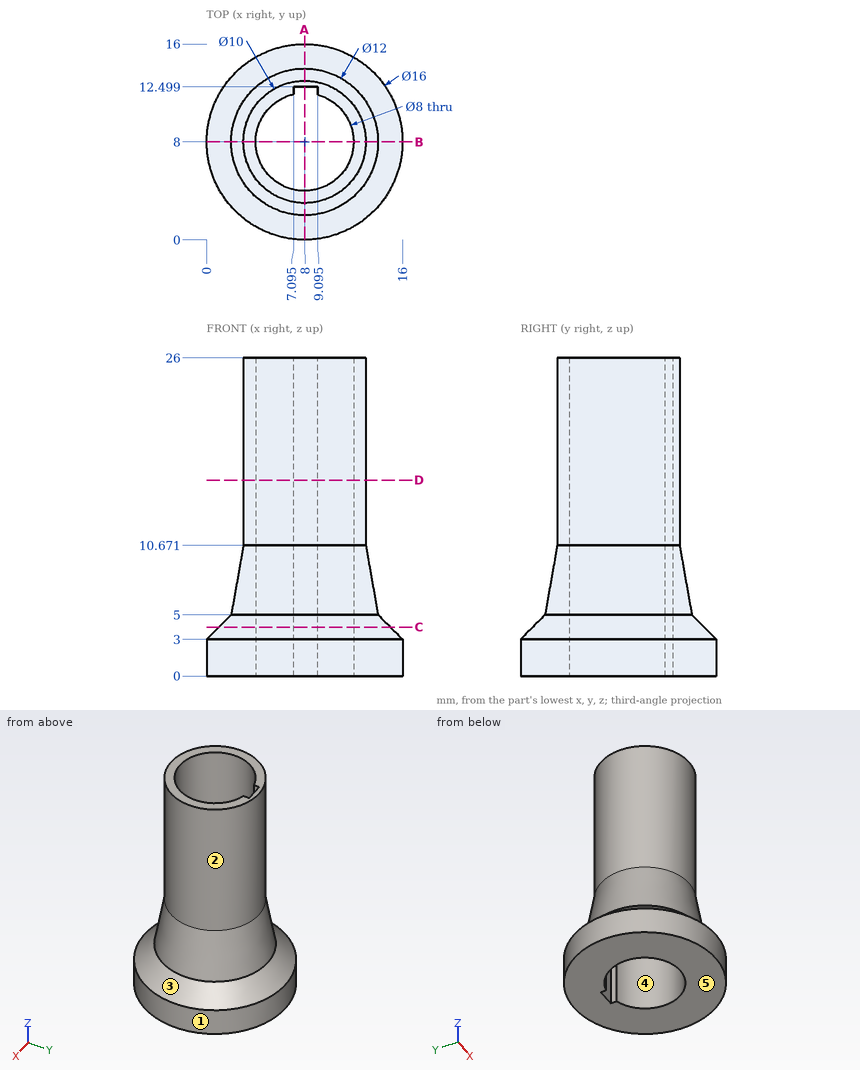
Design review of the part shown in the three views and the two pictorial views. Dimensions are in mm from the part's minimum x, y and z. A direction names the side the tool comes from. Round coordinates to 2 decimals unless told otherwise and drop trailing zeros. Order: outer loops, then holes, each group sorted by start corner. A loop starts at its lowest first (then second) coordinate and runs counter-clockwise, first axis right, second up. Notation, with made-up numbers: (-39, 17) -> (-19, 17) arc R28 cw to (-19, 50) -> close; hole circle Ø9 at (44, -26.75). An arc over 180 degrees is marked (long way). Write item = value, one per line. Start each with the question number.
1) Insertion check: pin 1 (0.5 mm diameter, centred on y = 12.5, z = 18, fed in from -X) (1 decimal); pin 2 (1 mm diameter, centred on y = 3.5, z = 7.5, fed in from -X) (1 decimal); pin 3 (6 mm diameter, centred on x = 12, z = 12.5, fed in from +Y); pin 4 (3 mm diameter, centred on x = 8.5, y = 8.5, fed in from -Z). Each pin has a flat end and moves straight along its axis. Give the tip position at first contact, or say it passes through.
2) Take a section at D-D on z = 16. State the section outline as (x, y) points (1 decimal), plus the area to 3 significant figures.
3) Take a section at B-B on y = 8. State the section outline as (x, z) points.
4) To check wall thickness, follow line 1 (Y direction, x = 10.75, z = 21) (1 decimal); line 2 (Y direction, x = 9, z = 10.5); line 3 (X direction, y = 12, z = 13) (1 decimal). State the ranges of each line that lie inside material, in increasing order. Write a range as from..to.
5) Take a section at C-C on z = 4. State the section outline as (x, y) points (1 decimal).
6) The part is to be moulded in two halves that separate along X. For the marked faces 3, 4 and 5, say which applies: +X half, -X half, draft (parallel to the pull), parting line (faces both ways), or undercut.
7) Take a section at A-A on x = 8. State the section outline as (y, z) points.
8) Tool access review of the marked faces 1 and 2: name each direction out of +Z, -Z, +X, -X, +Y, -Y from which nothing blocks a thin tool from reaching the whole face with its end or side.
Verdict:
q1.pin_1 = 5.4
q1.pin_2 = 4.1
q1.pin_3 = 12.9
q1.pin_4 = through
q2.outline = circle Ø10 at (8, 8); hole (7.1, 11.9) arc R4 ccw (long way) to (9.1, 11.8) -> (9.1, 12.5) -> (7.1, 12.5) -> close
q2.area = 27.2 mm2
q3.outline = (0, 0) -> (4, 0) -> (4, 26) -> (3, 26) -> (3, 10.67) -> (2, 5) -> (0, 3) -> close; (12, 0) -> (16, 0) -> (16, 3) -> (14, 5) -> (13, 10.67) -> (13, 26) -> (12, 26) -> close
q4.line_1 = 3.8..5.1, 10.9..12.2
q4.line_2 = 3.07..4.13, 12.5..12.93
q4.line_3 = 5..7.1, 9.1..11
q5.outline = circle Ø14 at (8, 8); hole (7.1, 11.9) arc R4 ccw (long way) to (9.1, 11.8) -> (9.1, 12.5) -> (7.1, 12.5) -> close
q6.face_3 = parting line
q6.face_4 = undercut
q6.face_5 = draft
q7.outline = (0, 0) -> (4, 0) -> (4, 26) -> (3, 26) -> (3, 10.67) -> (2, 5) -> (0, 3) -> close; (12.5, 0) -> (16, 0) -> (16, 3) -> (14, 5) -> (13, 10.67) -> (13, 26) -> (12.5, 26) -> close
q8.face_1 = +Z, -Z
q8.face_2 = +Z
